from build123d import *

# Parameters (mm, degrees)
F0_R     = 9.525
F1_DEPTH = 44.45
F2_R     = 6.34999
F4_DEPTH = 12.7
F5_R     = 9.525


# Not quite as in the source:
# - a fillet or chamfer is up to 0.001 mm smaller than in the source, because OpenCascade refuses the exact size


with BuildPart() as f1:
    # F0 (on Top) → F1 (new body)
    with BuildSketch(Plane.XY):
        with BuildLine():
            ThreePointArc((0, 19.05), (-13.4703841816, -13.4703841816), (19.05, 0))
            Line((19.05, 0), (19.05, 6.35))
            Line((19.05, 6.35), (17.9605122421, 6.35))
            ThreePointArc((17.9605122421, 6.35), (10.9985226281, 15.5542598667), (0, 19.05))
        make_face()
        Circle(F0_R, mode=Mode.SUBTRACT)
        with BuildLine():
            Line((38.1, 19.05), (0, 19.05))
            ThreePointArc((0, 19.05), (10.9985226281, 15.5542598667), (17.9605122421, 6.35))
            Line((17.9605122421, 6.35), (19.05, 6.35))
            Line((19.05, 6.35), (38.1, 6.35))
            Line((38.1, 6.35), (88.9, 6.35))
            Line((88.9, 6.35), (88.9, 19.05))
            Line((88.9, 19.05), (38.1, 19.05))
        make_face()
    extrude(amount=F1_DEPTH)

    # F2 (radius 6.35 in the source; OpenCascade refuses exactly that, so slightly less here)
    f2_edges = [f1.edges().sort_by_distance(p)[0] for p in [
        (19.05, 6.35, 22.225),
    ]]
    fillet(f2_edges, radius=F2_R)

    # F3 (on face) → F4 (cut)
    with BuildSketch(Plane.XZ.offset(-6.35)):
        with BuildLine():
            Line((88.9, 14.2875), (88.9, 30.1625))
            Line((88.9, 30.1625), (38.1, 30.1625))
            ThreePointArc((38.1, 30.1625), (43.7126600757, 27.8376600757), (46.0375, 22.225))
            ThreePointArc((46.0375, 22.225), (43.7126600757, 16.6123399243), (38.1, 14.2875))
            Line((38.1, 14.2875), (88.9, 14.2875))
        make_face()
        with BuildLine():
            ThreePointArc((46.0375, 22.225), (43.7126600757, 27.8376600757), (38.1, 30.1625))
            Line((38.1, 30.1625), (38.1, 22.225))
            Line((38.1, 22.225), (38.1, 14.2875))
            ThreePointArc((38.1, 14.2875), (43.7126600757, 16.6123399243), (46.0375, 22.225))
        make_face()
        with BuildLine():
            Line((38.1, 22.225), (38.1, 30.1625))
            ThreePointArc((38.1, 30.1625), (30.1625, 22.225), (38.1, 14.2875))
            Line((38.1, 14.2875), (38.1, 22.225))
        make_face()
    extrude(amount=-F4_DEPTH, mode=Mode.SUBTRACT)

    # F5
    f5_edges = [f1.edges().sort_by_distance(p)[0] for p in [
        (88.9, 12.7, 44.45),
        (88.9, 12.7, 0),
    ]]
    fillet(f5_edges, radius=F5_R)


solid = f1.part
Could you check a few things on this model? Use its own coordinates, in mm. A direction names the side the tool comes from. Coordinates: 2 decimals unless noted, no trailing zeros. Order: outer loops, then holes, each group sorted by start corner. A loop starts at its lowest first (then second) coordinate and runs counter-clockwise, first axis right, second up. Notation, with made-up numbers: (72, 69.25) -> (121, 69.25) arc R21 ccw to (121, 99.25) -> close; hole circle Ø8 at (31, -22). An arc over 180 degrees is marked (long way). One line per item, written item: value. Start each with the question number.
1) Imagine slicing it at A-A on x = 74.5. List the corners of the cut face in (y, z) for me, plus the area to 3 significant figures.
2) If I drill on L1, parallel to Y at x = 0, z = 28 (3 decimals); L2, parallel to Z at x = 63, y = 15.5; L3, parallel to Y at x = 67.5, z = 34.5, over which ranges is the centre line in solid material (lowest first)? Write a range as [from, to].
3) I'm going to push flat-ended pins straight in: pin 1 (13.5 mm diameter, centred on x = 63, z = 12.5, fed in from -Y); pin 2 (12 mm diameter, centred on y = 7, z = 16, fed in from +X); pin 3 (6 mm diameter, centred on y = -2, z = 7.5, fed in from +X); pin 4 (8 mm diameter, centred on y = -2.5, z = 16, fed in from +X). Where does each tip first touch, or does it pass through?
4) Which directions (+Z, -Z, +X, -X, +Y, -Y) give clear straight access to the entire face, cutting with the end or side of a thin tool? Please do faces 5 (the flat face through (57, 6.35, 12)), 6 (the flat face through (63, 13, 14.288)), 7 (the cylindrical face through (-7.559, -5.796, 21.914)).
5) We'd pull the mould along Z, two halves only. Please class faces 1 (the flat face through (64, 13, 30.162)), 2 (the flat face through (45, 19.05, 12)), 3 (the cylindrical face through (30.164, 12.611, 22.4)), 4 (the cylindrical face through (86.04, 12.79, 2.72)): +Z half, -Z half, draft (parallel to the pull), parting line (faces both ways), or undercut.
Answer list:
1. outline: (6.35, 0) -> (19.05, 0) -> (19.05, 14.29) -> (6.35, 14.29) -> close; (6.35, 30.16) -> (19.05, 30.16) -> (19.05, 44.45) -> (6.35, 44.45) -> close
1. area: 363 mm2
2. L1: y = [-19.05, -9.525], [9.525, 19.05]
2. L2: z = [0, 14.29], [30.16, 44.45]
2. L3: y = [6.35, 19.05]
3. pin 1: stops at y = 6.35
3. pin 2: stops at x = 88.9
3. pin 3: stops at x = 19.13
3. pin 4: stops at x = 19.23
4. face 5: +Z, -Z, +X, -Y
4. face 6: +X, +Y, -Y
4. face 7: +Z, -Z
5. face 1: undercut
5. face 2: draft
5. face 3: undercut
5. face 4: -Z half
